Could you check a few things on this model? Use its own coordinates, in mm. A direction names the side the tool comes from. Give positions to 0.01 mm unless a question says otherwise; leave off trailing zeros. Order: outer loops, then holes, each group sorted by start corner. A loop starts at its lowest first (then second) coordinate and runs counter-clockwise, first axis right, second up.
(1) Imagine slicing it at B-B, the plane z = 12. Write out the boundary of the cut face in (x, y) (3 decimals), then the cut area to 3 significant figures.
(2) Imagine slicing it at A-A, the plane x = -1. Write out the boundary of the cut face in (y, z) (3 decimals).
(3) Will these pins go through, and if not, where does the flat tip stop? pin 1 (1.2 mm diameter, centred on y = 6, z = 1, fed in from +X); pin 2 (7 mm diameter, centred on x = 2.5, z = 4.5, fed in from +Y); pin 3 (5 mm diameter, centred on y = 10.5, z = 3.5, fed in from -X).
(4) On a 3-axis mill with a long thin cutter (end or side, diameter ignored), from which of +Z, -Z, +X, -X, +Y, -Y can I reach the whole of each face in a straight line? I mean faces 1 (the cylindrical face through (-5.715, 6.479, 2.199)), 2 (the flat face through (0, 0, 13.45)), 3 (the flat face through (4, 7, 1)). Say none if no direction works.
(5) If we mould it in two halves opening along X, with no side actions, what happens to faces 4 (the cylindrical face through (-8.274, -4.43, 7.161)), 5 (the flat face through (0, 5, 6)), 6 (the cylindrical face through (-5.865, 0.07, 13.149))? For each: released by +X, released by -X, zero draft, split by the parting line, or undercut.
(6) Imagine slicing it at C-C, the plane y = -1.5. Write out the boundary of the cut face in (x, z) (3 decimals).
(7) If I drill on probe 1 along Z at (x, y) = (4.75, -1.75) (3 decimals); probe 2 along X at (y, z) = (-2.25, 9.25) (3 decimals); probe 3 along Z at (x, y) = (-3.5, 7.25), over which ranges is the centre line in solid material (lowest first)?
(8) Imagine slicing it at D-D, the plane z = 2.75. Write out the boundary of the cut face in (x, y) (3 decimals).
from build123d import *

# Parameters (mm, degrees)
SKETCH042_W     = 17.75
SKETCH042_H     = 10
PAD023_DEPTH    = 16.625
SKETCH043_W     = 12.3
SKETCH043_H     = 6.5
POCKET020_DEPTH = 10
FILLET013_R     = 1
FILLET014_R     = 2.5
FILLET015_R     = 2
FILLET016_R     = 2
SKETCH044_R     = 1.6
PAD024_DEPTH    = 2.5
FILLET017_R     = 1


with BuildPart() as part:
    # Sketch042 → Pad023 (new body)
    with BuildSketch(Plane.XY):
        Rectangle(SKETCH042_W, SKETCH042_H)
    extrude(amount=PAD023_DEPTH)

    # Sketch043 (on Face3 of Pad023) → Pocket020 (cut)
    with BuildSketch(Plane.XZ.offset(5)):
        with Locations((0, 10.2)):
            Rectangle(SKETCH043_W, SKETCH043_H)
    extrude(amount=-POCKET020_DEPTH, mode=Mode.SUBTRACT)

    # Fillet013
    fillet013_edges = [part.edges().sort_by_distance(p)[0] for p in [
        (-6.15, 0, 13.45),
        (6.15, 0, 13.45),
        (6.15, 0, 6.95),
        (-6.15, 0, 6.95),
    ]]
    fillet(fillet013_edges, radius=FILLET013_R)

    # Fillet014
    fillet014_edges = [part.edges().sort_by_distance(p)[0] for p in [
        (8.875, 0, 16.625),
        (-8.875, 0, 16.625),
    ]]
    fillet(fillet014_edges, radius=FILLET014_R)

    # Fillet015
    fillet015_edges = [part.edges().sort_by_distance(p)[0] for p in [
        (8.875, 5, 7.0625),
        (-8.875, 5, 7.0625),
    ]]
    fillet(fillet015_edges, radius=FILLET015_R)

    # Fillet016
    fillet016_edges = [part.edges().sort_by_distance(p)[0] for p in [
        (0, -5, 16.625),
    ]]
    fillet(fillet016_edges, radius=FILLET016_R)

    # Sketch044 → Pad024 (join)
    with BuildSketch(Plane.XY):
        with BuildLine():
            Line((-6, 8), (-6, 0))
            Line((-6, 0), (4, 0))
            Line((4, 8), (4, 0))
            ThreePointArc((4, 8), (-1, 13), (-6, 8))
        make_face()
        with Locations((-1, 8)):
            Circle(SKETCH044_R, mode=Mode.SUBTRACT)
    extrude(amount=PAD024_DEPTH)

    # Fillet017
    fillet017_edges = [part.edges().sort_by_distance(p)[0] for p in [
        (-6, 6.5, 2.5),
        (-1, 13, 2.5),
        (4, 6.5, 2.5),
    ]]
    fillet(fillet017_edges, radius=FILLET017_R)


solid = part.part
Answer block:
1. outline: (-8.875, -3) arc R2 ccw to (-6.875, -5) - (-6.15, -5) - (-6.15, 5) - (-6.875, 5) arc R2 ccw to (-8.875, 3) - close; (6.15, -5) - (6.875, -5) arc R2 ccw to (8.875, -3) - (8.875, 3) arc R2 ccw to (6.875, 5) - (6.15, 5) - close
1. area: 51.1 mm2
2. outline: (-5, 0) - (6.4, 0) - (6.4, 2.5) - (5, 2.5) - (5, 6.95) - (-5, 6.95) - close; (-5, 13.45) - (5, 13.45) - (5, 14.625) arc R2 ccw to (3, 16.625) - (-3, 16.625) arc R2 ccw to (-5, 14.625) - close; (9.6, 0) - (13, 0) - (13, 1.5) arc R1 ccw to (12, 2.5) - (9.6, 2.5) - close
3. pin 1: stops at x = 4
3. pin 2: stops at y = 12.79
3. pin 3: stops at x = -5.92
4. face 1: +Z, -X, +Y
4. face 2: +Y, -Y
4. face 3: +Z, -Z, +X, +Y
5. face 4: released by -X
5. face 5: zero draft
5. face 6: undercut
6. outline: (-8.875, 0) - (8.875, 0) - (8.875, 14.125) arc R2.5 ccw to (6.375, 16.625) - (-6.375, 16.625) arc R2.5 ccw to (-8.875, 14.125) - close; hole (-6.15, 7.95) arc R1 ccw to (-5.15, 6.95) - (5.15, 6.95) arc R1 ccw to (6.15, 7.95) - (6.15, 12.45) arc R1 ccw to (5.15, 13.45) - (-5.15, 13.45) arc R1 ccw to (-6.15, 12.45) - close
7. probe 1: z = 0 to 6.95, 13.45 to 16.625
7. probe 2: x = -8.875 to -6.15, 6.15 to 8.875
7. probe 3: z = 0 to 2.5
8. outline: (-8.875, -3) arc R2 ccw to (-6.875, -5) - (6.875, -5) arc R2 ccw to (8.875, -3) - (8.875, 3) arc R2 ccw to (6.875, 5) - (-6.875, 5) arc R2 ccw to (-8.875, 3) - close
